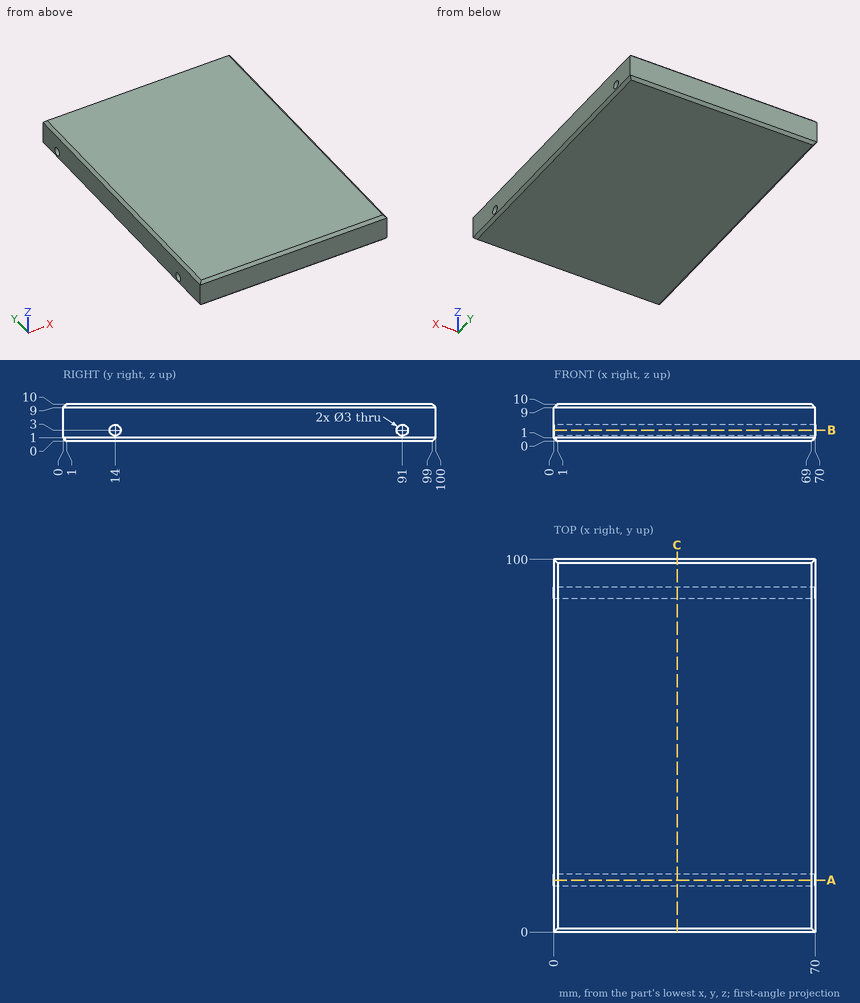
For this review, use the dimensioned drawing (mm, ordinates from the lowest corner) and the shaded views. Coordinates: 2 decimals unless noted, no trailing zeros. Order: outer loops, then holes, each group sorted by start corner. A loop starts at its lowest first (then second) coordinate and runs counter-clockwise, first axis right, second up. Notation, with made-up numbers: (40.5, 46.5) - (60.5, 46.5) arc R31 cw to (60.5, 80.5) - close; hole circle Ø7 at (-27.75, -1). An arc over 180 degrees is marked (long way). Use one line per item in the form item = value.
Q1. Consider section B-B (z = 3). Give the boundary of the cut face in (x, y).
Checked values:
outline = (0, 0) - (70, 0) - (70, 12.5) - (0, 12.5) - close; (0, 15.5) - (70, 15.5) - (70, 89.5) - (0, 89.5) - close; (0, 92.5) - (70, 92.5) - (70, 100) - (0, 100) - close
Q2. For probe 1 along Y at (x, z) = (17.5, 2.75); probe 2 along Z at (x, y) = (22.5, 14); probe 3 along X at (y, z) = (73, 0.5), list the stretches that pass through material, from the lowest coordinate up. Write a range as from..to.
Checked values:
probe_1 = 0..12.52, 15.48..89.52, 92.48..100
probe_2 = 0..1.5, 4.5..10
probe_3 = 0.5..69.5
Q3. For P1, Ø2.5, axis at y = 14, z = 3, coming from the -X side, flat-tipped, find the tip position at first contact; note if it passes through.
Checked values:
P1 = through
Q4. Consider section C-C (x = 33). Give the boundary of the cut face in (y, z).
Checked values:
outline = (0, 1) - (1, 0) - (99, 0) - (100, 1) - (100, 9) - (99, 10) - (1, 10) - (0, 9) - close; hole circle Ø3 at (14, 3); hole circle Ø3 at (91, 3)
Q5. Consider section A-A (y = 14). Give the boundary of the cut face in (x, z), then the cut area to 3 significant figures.
Checked values:
outline = (0, 1) - (1, 0) - (69, 0) - (70, 1) - (70, 1.5) - (0, 1.5) - close; (0, 4.5) - (70, 4.5) - (70, 9) - (69, 10) - (1, 10) - (0, 9) - close
area = 488 mm2
